Here's how the part is built. I have some questions about the finished solid (model axes, mm). Face numbers are marked on the shaded views. A direction names the side the tool comes from. Round coordinates to 2 decimals unless told otherwise and drop trailing zeros. Order: outer loops, then holes, each group sorted by start corner. A loop starts at its lowest first (then second) coordinate and runs counter-clockwise, first axis right, second up. Notation, with made-up numbers: (9.5, 76) -> (16.5, 76) arc R35 ccw to (16.5, 111) -> close; hole circle Ø8 at (73.5, 30.25). An arc over 180 degrees is marked (long way). Use a Markdown table: item, result. Add a question column.
(1) I want a section at A-A, the plane x = 0. Please give me the cut outline in (y, z).
(2) On a 3-axis mill with a long thin cutter (end or side, diameter ignored), from which of +Z, -Z, +X, -X, +Y, -Y can I reach the whole of each face in a straight line? I mean the marked faces 1, 2 and 3. Say none if no direction works.
(3) I'm going to push a flat-ended pin straight in: P1, Ø1, axis at y = 1.5, z = 5.5, coming from the +X side. Where does the tip first touch, or does it pass through?
(4) I want a section at D-D, the plane z = 7. Please give me the cut outline in (x, y).
(5) I want a section at C-C, the plane z = 3.5. Please give me the cut outline in (x, y), then the cut area to 3 significant figures.
(6) If I drill on probe 1 along Y at (x, z) = (0, 3.8); probe 2 along Z at (x, y) = (-0.55, 0.05); probe 3 along X at (y, z) = (0.25, 2), over which ranges is the centre line in solid material (lowest first)?
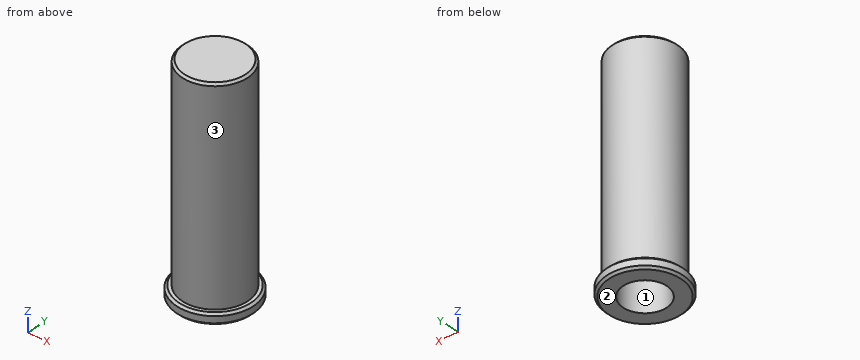
from build123d import *

# Parameters (mm, degrees)
SKETCH_1_R          = 1.5
EXTRUDE_1_DEPTH     = 10
SKETCH_2_R          = 1.75
EXTRUDE_2_DEPTH     = 0.5
CHAMFER_1_SIZE      = 0.1
SKETCH_3_R          = 1
CUT_EXTRUDE_1_DEPTH = 5


with BuildPart() as part:
    # 草图1 → 凸台-拉伸1 (new body)
    with BuildSketch(Plane.XY):
        Circle(SKETCH_1_R)
    extrude(amount=EXTRUDE_1_DEPTH)

    # 草图2 → 凸台-拉伸2 (add)
    with BuildSketch(Plane(origin=(0, 0, 0), x_dir=(-1, 0, 0), z_dir=(0, 0, -1))):
        Circle(SKETCH_2_R)
    extrude(amount=-EXTRUDE_2_DEPTH)

    # 倒角1
    chamfer_1_edges = [part.edges().sort_by_distance(p)[0] for p in [
        (-1.5, 0, 10),
        (1.75, 0, 0.5),
        (1.75, 0, 0),
    ]]
    chamfer(chamfer_1_edges, length=CHAMFER_1_SIZE)

    # 草图3 → 切除-拉伸1 (cut)
    with BuildSketch(Plane(origin=(0, 0, 0), x_dir=(-1, 0, 0), z_dir=(0, 0, -1))):
        Circle(SKETCH_3_R)
    extrude(amount=-CUT_EXTRUDE_1_DEPTH, mode=Mode.SUBTRACT)


solid = part.part
Taken from the geometry:
| question | item | result |
|---|---|---|
| 1 | outline | (-1.75, 0.1) -> (-1.65, 0) -> (-1, 0) -> (-1, 5) -> (1, 5) -> (1, 0) -> (1.65, 0) -> (1.75, 0.1) -> (1.75, 0.4) -> (1.65, 0.5) -> (1.5, 0.5) -> (1.5, 9.9) -> (1.4, 10) -> (-1.4, 10) -> (-1.5, 9.9) -> (-1.5, 0.5) -> (-1.65, 0.5) -> (-1.75, 0.4) -> close |
| 2 | face 1 | -Z |
| 2 | face 2 | -Z, +X, -X, +Y, -Y |
| 2 | face 3 | +Z |
| 3 | P1 | stops at x = 1.12 |
| 4 | outline | circle Ø3 at (0, 0) |
| 5 | outline | circle Ø3 at (0, 0); hole circle Ø2 at (0, 0) |
| 5 | area | 3.93 mm2 |
| 6 | probe 1 | y = -1.5 to -1, 1 to 1.5 |
| 6 | probe 2 | z = 5 to 10 |
| 6 | probe 3 | x = -1.48 to -0.97, 0.97 to 1.48 |
